from build123d import *

# Parameters (mm, degrees)
SKETCH1_W               = 19.05
SKETCH1_H               = 19.05
SKETCH1_W_2             = 15.748
SKETCH1_H_2             = 15.748
BOSS_EXTRUDE1_DEPTH     = 28.575
CUT_EXTRUDE2_DEPTH      = 36.639286609
CUT_EXTRUDE2_DEPTH_BACK = 36.639286609
SKETCH3_R               = 4.064
CUT_EXTRUDE4_DEPTH      = 36.639286609
CUT_EXTRUDE4_DEPTH_BACK = 36.639286609
SKETCH4_W               = 15.748
SKETCH4_H               = 15.24
FILLET2_R               = 6.35
CUT_EXTRUDE5_START      = -10.431366523
CUT_EXTRUDE5_DEPTH      = 20.862732946


# Read off the part's stored shape, not the designer's step: Cut-Extrude5
with BuildPart() as part:
    # Sketch1 → Boss-Extrude1 (new body)
    with BuildSketch(Plane.XY):
        Rectangle(SKETCH1_W, SKETCH1_H)
        Rectangle(SKETCH1_W_2, SKETCH1_H_2, mode=Mode.SUBTRACT)
    extrude(amount=BOSS_EXTRUDE1_DEPTH)

    # Sketch3 → Cut-Extrude2 (cut, two sides: drawn at the far end of the back side and taken through both)
    with BuildSketch(Plane(origin=(9.525, 0, 0), x_dir=(0, 0, -1), z_dir=(1, 0, 0)).offset(-CUT_EXTRUDE2_DEPTH_BACK)):
        with Locations(Location((-20.6375, 0, 0), (0, 0, 90))):
            Circle(SKETCH3_R)
    extrude(amount=CUT_EXTRUDE2_DEPTH + CUT_EXTRUDE2_DEPTH_BACK, mode=Mode.SUBTRACT)

    # Sketch4 → Cut-Extrude4 (cut, two sides: drawn at the far end of the back side and taken through both)
    with BuildSketch(Plane.XZ.offset(9.525).offset(-CUT_EXTRUDE4_DEPTH_BACK)):
        with Locations((0, 20.955)):
            Rectangle(SKETCH4_W, SKETCH4_H)
    extrude(amount=CUT_EXTRUDE4_DEPTH + CUT_EXTRUDE4_DEPTH_BACK, mode=Mode.SUBTRACT)

    # Fillet2
    fillet2_edges = [part.edges().sort_by_distance(p)[0] for p in [
        (-8.6995, -9.525, 28.575),
        (8.6995, -9.525, 28.575),
        (-8.6995, 9.525, 28.575),
        (8.6995, 9.525, 28.575),
    ]]
    fillet(fillet2_edges, radius=FILLET2_R)

    # Cut-Extrude5 outline → Cut-Extrude5 (cut)
    with BuildSketch(Plane(origin=(0, 0, 0), x_dir=(0.9949685182509123, 0.10018806161207, 0), z_dir=(0.10018806161207001, -0.9949685182509123, 0)).offset(CUT_EXTRUDE5_START)):
        with BuildLine():
            add(Edge.make_bspline(
                [(-9.477075136, 0), (0, 10.800334816), (9.477075136, 0)],
                knots=[5.435123228, 5.435123228, 5.435123228, 7.131247386, 7.131247386, 7.131247386], degree=2, weights=[1, 0.661437828, 1]))
            Line((-9.477075136, 0), (9.477075136, 0))
        make_face()
    extrude(amount=CUT_EXTRUDE5_DEPTH, mode=Mode.SUBTRACT)


solid = part.part
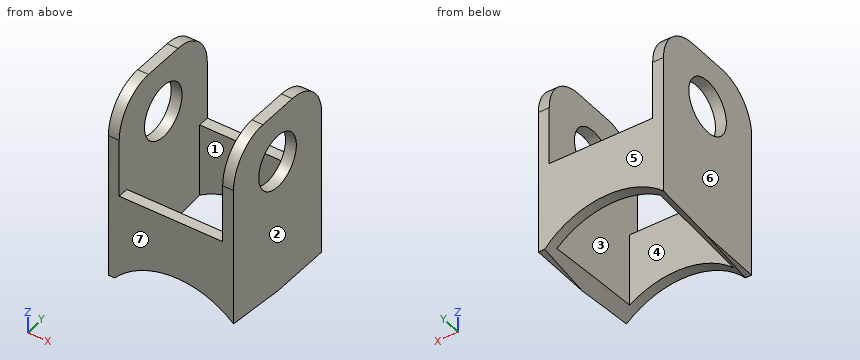
Read the model definition and answer for the solid it produces. Units are mm, in the model's axes. Face numbers are marked on the shaded views. A direction names the side the tool comes from. Give positions to 0.01 mm unless a question says otherwise; leave off trailing zeros. Loops run counter-clockwise (first coordinate to the right, second up) from the corner with the lowest first, then second, coordinate; pieces in that order, holes last. Notation, with made-up numbers: (-12.75, 26) -> (5.25, 26) arc R21 cw to (5.25, 55) -> close; hole circle Ø6 at (3, 49.25). An arc over 180 degrees is marked (long way). Answer as CSV lines item,"result".
Item 1: Consider line 1 (Y direction, x = -1.75, z = 11.75) (3 decimals); line 2 (Z direction, x = 8.9, y = 0) (1 decimal). Determine where each line is inside the solid, lowest interval first. Write a range as [from, to].
Returned:
line 1,"y = [-9.525, -7.874], [7.874, 9.525]"
line 2,"z = [0.7, 16.6], [24.7, 28.6]"
Item 2: Find section A-A on z = 6.5. Give the vertices of the cut face in (x, y) (3 decimals), plus the area to 3 significant figures.
Returned:
outline,"(-9.525, -9.525) -> (9.525, -9.525) -> (9.525, 9.525) -> (-9.525, 9.525) -> close; hole (-7.874, -7.874) -> (7.874, -7.874) -> (7.874, 7.874) -> (-7.874, 7.874) -> close"
area,"115 mm²"
Item 3: For the marked faces 1, 2 and 3, determine the directions among +Z, -Z, +X, -X, +Y, -Y from which every point of the face is accessible in a straight line to the end or side of a thin tool.
Returned:
face 1,"+Z, -Z"
face 2,"+Z, -Z, +X, +Y, -Y"
face 3,"+Z"
Item 4: Each of these flat-tipped pins is pushed along its axis until it touches: pin 1 (1.8 mm diameter, centred on x = 2.5, y = -8.5, fed in from +Z) (3 decimals); pin 2 (1 mm diameter, centred on x = -7, y = -5, fed in from -Z). Where does it stop, or does it pass through?
Returned:
pin 1,"stops at z = 13.335"
pin 2,"passes through"
Item 5: Determine the mould class of the marked faces 4, 5, 6 and 7 for opening direction Y: +Y half, -Y half, draft (parallel to the pull), parting line (faces both ways), or undercut.
Returned:
face 4,"undercut"
face 5,"+Y half"
face 6,"draft"
face 7,"-Y half"
Item 6: Find section B-B on y = 1. State how many separate pieces and enclosed holes the cut face has, plus the area to 3 significant figures.
Returned:
separate pieces,"4"
enclosed holes,"0"
area,"65.6 mm²"
